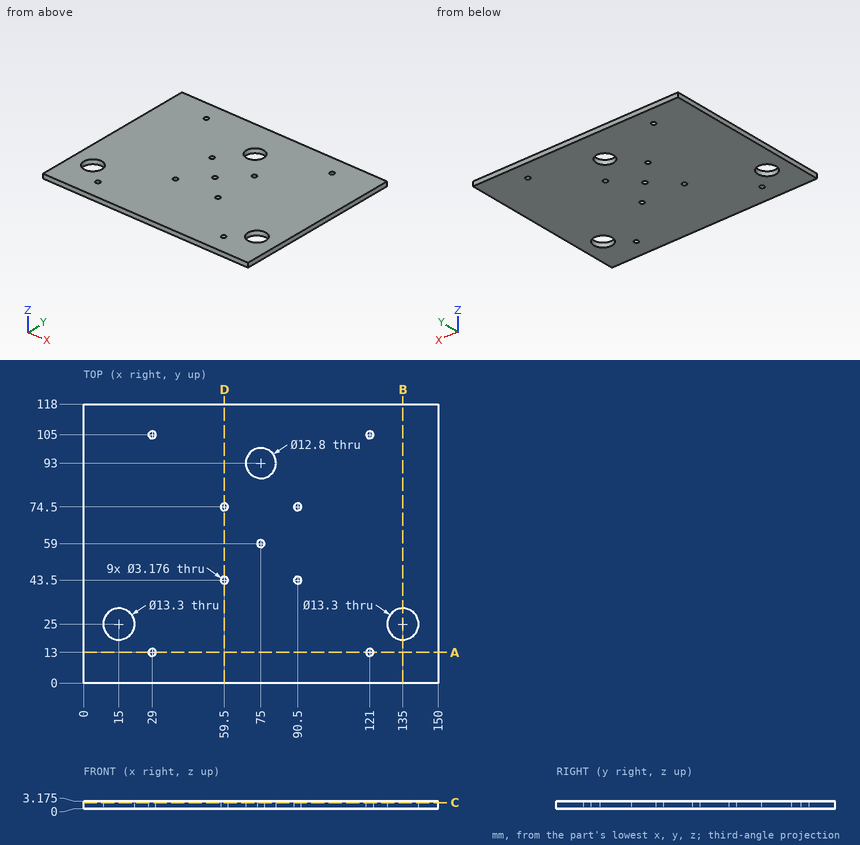
Geometry check sheet. Reference: drawing and pictorial views, mm from the part's lowest x, y, z. Round coordinates to 2 decimals unless told otherwise and drop trailing zeros. Order: outer loops, then holes, each group sorted by start corner. A loop starts at its lowest first (then second) coordinate and runs counter-clockwise, first axis right, second up. Notation, with made-up numbers: (23.25, 30.5) - (45.25, 30.5) arc R17 cw to (45.25, 39.5) - close; hole circle Ø11 at (33.5, 10.25). An arc over 180 degrees is marked (long way). Use a Markdown table: item, result. Add a question column.
1) Thickness scan on line 1 along Y through (x, z) = (121, 2.1); line 2 along Y through (x, z) = (75, 1.6); line 3 along X through (y, z) = (105, 1.1). Record the ranges inside material, lowest first.
2) Section check C-C (z = 2.6). Count the separate pieces of the cut face and the enclosed holes in it, then the cut area to 3 significant figures.
3) Section check A-A (y = 13). Record the cut outline in (x, z) (3 decimals).
4) Section check B-B (x = 135). Record the cut outline in (y, z) (3 decimals).
5) Section check D-D (x = 59.5). Record the cut outline in (y, z) (3 decimals), then the cut area to 3 significant figures.
Established:
| question | item | result |
|---|---|---|
| 1 | line 1 | 0 to 11.41, 14.59 to 103.41, 106.59 to 118 |
| 1 | line 2 | 0 to 57.41, 60.59 to 86.6, 99.4 to 118 |
| 1 | line 3 | 0 to 27.41, 30.59 to 119.41, 122.59 to 150 |
| 2 | separate pieces | 1 |
| 2 | enclosed holes | 12 |
| 2 | area | 17,200 mm2 |
| 3 | outline | (0, 0) - (27.412, 0) - (27.412, 3.175) - (0, 3.175) - close; (30.588, 0) - (119.412, 0) - (119.412, 3.175) - (30.588, 3.175) - close; (122.588, 0) - (150, 0) - (150, 3.175) - (122.588, 3.175) - close |
| 4 | outline | (0, 0) - (18.35, 0) - (18.35, 3.175) - (0, 3.175) - close; (31.65, 0) - (118, 0) - (118, 3.175) - (31.65, 3.175) - close |
| 5 | outline | (0, 0) - (41.912, 0) - (41.912, 3.175) - (0, 3.175) - close; (45.088, 0) - (72.912, 0) - (72.912, 3.175) - (45.088, 3.175) - close; (76.088, 0) - (118, 0) - (118, 3.175) - (76.088, 3.175) - close |
| 5 | area | 354 mm2 |
